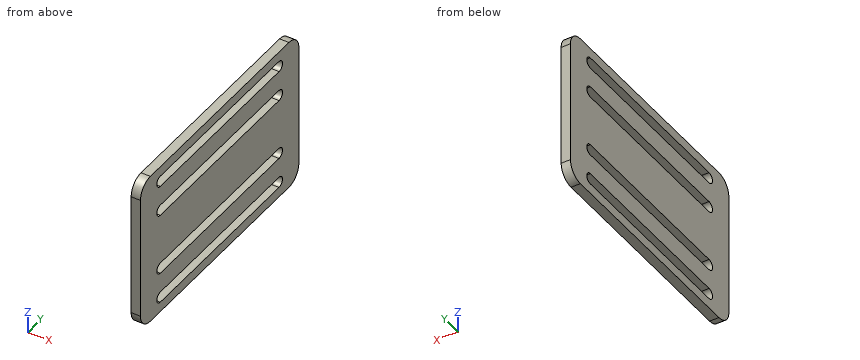
from build123d import *

# Parameters (mm, degrees)
SKETCH_1_W      = 50
SKETCH_1_H      = 80
SKETCH_1_R      = 1.75
EXTRUDE_1_DEPTH = 3
FILLET_1_R      = 5


with BuildPart() as part:
    # 草图1 → 凸台-拉伸1 (new body)
    # profile 1 of 4: a face of its own
    with BuildSketch(Plane(origin=(0, 0, 0), x_dir=(0, 0, -1), z_dir=(1, 0, 0))):
        Rectangle(SKETCH_1_W, SKETCH_1_H)
        with BuildLine():
            Line((-21.75, -30), (-21.75, 30))
            ThreePointArc((-21.75, 30), (-20, 31.75), (-18.25, 30))
            Line((-18.25, 30), (-18.25, -30))
            ThreePointArc((-18.25, -30), (-20, -31.75), (-21.75, -30))
        make_face(mode=Mode.SUBTRACT)
        with BuildLine():
            Line((-11.75, -30), (-11.75, 30))
            ThreePointArc((-11.75, 30), (-10, 31.75), (-8.25, 30))
            Line((-8.25, 30), (-8.25, -30))
            ThreePointArc((-8.25, -30), (-10, -31.75), (-11.75, -30))
        make_face(mode=Mode.SUBTRACT)
        with BuildLine():
            Line((-1.75, -30), (-1.75, 30))
            ThreePointArc((-1.75, 30), (0, 31.75), (1.75, 30))
            Line((1.75, 30), (1.75, -30))
            ThreePointArc((1.75, -30), (0, -31.75), (-1.75, -30))
        make_face(mode=Mode.SUBTRACT)
        with BuildLine():
            Line((8.25, -30), (8.25, 30))
            ThreePointArc((8.25, 30), (10, 31.75), (11.75, 30))
            Line((11.75, 30), (11.75, -30))
            ThreePointArc((11.75, -30), (10, -31.75), (8.25, -30))
        make_face(mode=Mode.SUBTRACT)
        with BuildLine():
            Line((21.75, 30), (21.75, -30))
            ThreePointArc((21.75, -30), (20, -31.75), (18.25, -30))
            Line((18.25, -30), (18.25, 30))
            ThreePointArc((18.25, 30), (20, 31.75), (21.75, 30))
        make_face(mode=Mode.SUBTRACT)
    # profile 2 of 4: a face of its own
    with BuildSketch(Plane(origin=(0, 0, 0), x_dir=(0, 0, -1), z_dir=(1, 0, 0))):
        with BuildLine():
            ThreePointArc((1.75, 30), (0, 28.25), (-1.75, 30))
            Line((-1.75, 30), (-1.75, -30))
            ThreePointArc((-1.75, -30), (0, -28.25), (1.75, -30))
            Line((1.75, -30), (1.75, 30))
        make_face()
    # profile 3 of 4: a face of its own
    with BuildSketch(Plane(origin=(0, 0, 0), x_dir=(0, 0, -1), z_dir=(1, 0, 0))):
        with Locations((0, 30)):
            Circle(SKETCH_1_R)
    # profile 4 of 4: a face of its own
    with BuildSketch(Plane(origin=(0, 0, 0), x_dir=(0, 0, -1), z_dir=(1, 0, 0))):
        with Locations((0, -30)):
            Circle(SKETCH_1_R)
    extrude(amount=EXTRUDE_1_DEPTH)

    # 圆角1
    fillet_1_edges = [part.edges().sort_by_distance(p)[0] for p in [
        (1.5, -40, -25),
        (1.5, -40, 25),
        (1.5, 40, 25),
        (1.5, 40, -25),
    ]]
    fillet(fillet_1_edges, radius=FILLET_1_R)


solid = part.part
Geometry check sheet. Reference: the model listing, model coordinates, mm. Give positions to 0.01 mm unless a question says otherwise; leave off trailing zeros. Order: outer loops, then holes, each group sorted by start corner. A loop starts at its lowest first (then second) coordinate and runs counter-clockwise, first axis right, second up. Notation, with made-up numbers: (-29.75, -35) - (10.25, -35) arc R9 cw to (10.25, -23) - close; hole circle Ø5 at (-33.5, -3.5). An arc over 180 degrees is marked (long way). Use one line per item in the form item = value.
1) Material ranges on probe 1 along Z at (x, y) = (1.35, -17); probe 2 along Y at (x, z) = (2, -10.5); probe 3 along Y at (x, z) = (1.75, -11.5), recorded low to high. Write a range as from..to.
Working result:
probe_1 = -25..-21.75, -18.25..-11.75, -8.25..8.25, 11.75..18.25, 21.75..25
probe_2 = -40..-31.68, 31.68..40
probe_3 = -40..-30.9, 30.9..40
2) Sectioned sample at C-C (x = 2.1). Record the boundary of the cut face in (y, z), and give its area (3 significant figures).
Working result:
outline = (-40, -20) arc R5 ccw to (-35, -25) - (35, -25) arc R5 ccw to (40, -20) - (40, 20) arc R5 ccw to (35, 25) - (-35, 25) arc R5 ccw to (-40, 20) - close; hole (-30, -21.75) - (30, -21.75) arc R1.75 ccw to (30, -18.25) - (-30, -18.25) arc R1.75 ccw to start; hole (-30, -11.75) - (30, -11.75) arc R1.75 ccw to (30, -8.25) - (-30, -8.25) arc R1.75 ccw to start; hole (-30, 8.25) - (30, 8.25) arc R1.75 ccw to (30, 11.75) - (-30, 11.75) arc R1.75 ccw to start; hole (-30, 18.25) - (30, 18.25) arc R1.75 ccw to (30, 21.75) - (-30, 21.75) arc R1.75 ccw to start
area = 3,100 mm^2
3) Sectioned sample at A-A (z = -10). Record the boundary of the cut face in (x, y).
Working result:
outline = (0, -40) - (3, -40) - (3, -31.75) - (0, -31.75) - close; (0, 31.75) - (3, 31.75) - (3, 40) - (0, 40) - close
4) Sectioned sample at B-B (y = 16). Record the boundary of the cut face in (x, z).
Working result:
outline = (0, -25) - (3, -25) - (3, -21.75) - (0, -21.75) - close; (0, -18.25) - (3, -18.25) - (3, -11.75) - (0, -11.75) - close; (0, -8.25) - (3, -8.25) - (3, 8.25) - (0, 8.25) - close; (0, 11.75) - (3, 11.75) - (3, 18.25) - (0, 18.25) - close; (0, 21.75) - (3, 21.75) - (3, 25) - (0, 25) - close
